```python
from build123d import *

# Parameters (mm, degrees)
SM_BASE_FLANGE_1_DEPTH = 351
SKETCH_6_W             = 30
SKETCH_6_H             = 25
CUT_EXTRUDE_1_DEPTH    = 3
SKETCH_7_R             = 2.5
CUT_EXTRUDE_1299_DEPTH = 569.507695638
SKETCH_8_R             = 3
CUT_EXTRUDE_1710_DEPTH = 1.5
SKETCH_10_W            = 65
SKETCH_10_H            = 25
CUT_EXTRUDE_4_DEPTH    = 3
OTHER_START            = -361.5
OTHER_1_DEPTH          = 723
SKETCH_11_R            = 10
CUT_EXTRUDE_2693_DEPTH = 10
SKETCH_12_R            = 4
CUT_EXTRUDE_3148_DEPTH = 10
SKETCH_13_R            = 2.5
SKETCH_13_R_2          = 5.5
CUT_EXTRUDE_3688_DEPTH = 10
SKETCH_15_R            = 14.5
SKETCH_15_R_2          = 2.5
CUT_EXTRUDE_4428_DEPTH = 1.5
SKETCH_16_R            = 2.5
CUT_EXTRUDE_5_DEPTH    = 10
SKETCH_17_W            = 100
SKETCH_17_H            = 10
CUT_EXTRUDE_6_DEPTH    = 10


# Read off the part's stored shape, not the designer's step: Затупленный угол1
# Sheet-metal steps are written as plain solids
with BuildPart() as part:
    # Sketch 1 → Базовая кромка1 (new, symmetric)
    with BuildSketch(Plane.XY):
        with BuildLine():
            Line((360, -175), (360, -197))
            ThreePointArc((360, -197), (360.878679656, -199.121320344), (363, -200))
            Line((363, -200), (397, -200))
            ThreePointArc((397, -200), (399.121320344, -199.121320344), (400, -197))
            Line((400, -197), (400, -3))
            ThreePointArc((400, -3), (399.121320344, -0.878679656), (397, 0))
            Line((397, 0), (-397, 0))
            ThreePointArc((-397, 0), (-399.121320344, -0.878679656), (-400, -3))
            Line((-400, -3), (-400, -197))
            ThreePointArc((-400, -197), (-399.121320344, -199.121320344), (-397, -200))
            Line((-397, -200), (-363, -200))
            ThreePointArc((-363, -200), (-360.878679656, -199.121320344), (-360, -197))
            Line((-360, -197), (-360, -175))
            Line((-360, -175), (-361.5, -175))
            Line((-361.5, -175), (-361.5, -197))
            ThreePointArc((-361.5, -197), (-361.939339828, -198.060660172), (-363, -198.5))
            Line((-363, -198.5), (-397, -198.5))
            ThreePointArc((-397, -198.5), (-398.060660172, -198.060660172), (-398.5, -197))
            Line((-398.5, -197), (-398.5, -3))
            ThreePointArc((-398.5, -3), (-398.060660172, -1.939339828), (-397, -1.5))
            Line((-397, -1.5), (397, -1.5))
            ThreePointArc((397, -1.5), (398.060660172, -1.939339828), (398.5, -3))
            Line((398.5, -3), (398.5, -197))
            ThreePointArc((398.5, -197), (398.060660172, -198.060660172), (397, -198.5))
            Line((397, -198.5), (363, -198.5))
            ThreePointArc((363, -198.5), (361.939339828, -198.060660172), (361.5, -197))
            Line((361.5, -197), (361.5, -175))
            Line((361.5, -175), (360, -175))
        make_face()
    extrude(amount=SM_BASE_FLANGE_1_DEPTH, both=True)

    # Эскиз6 → Вырез-Вытянуть1 (cut)
    with BuildSketch(Plane(origin=(-360, 0, 0), x_dir=(0, 0, -1), z_dir=(1, 0, 0))):
        with Locations((-336, -187.5)):
            Rectangle(SKETCH_6_W, SKETCH_6_H)
        with Locations((336, -187.5)):
            Rectangle(SKETCH_6_W, SKETCH_6_H)
    cut_extrude_1 = extrude(amount=-CUT_EXTRUDE_1_DEPTH, mode=Mode.SUBTRACT)

    # Зеркальное отражение1: Вырез-Вытянуть1 across plane
    add(cut_extrude_1.mirror(Plane(origin=(0, 0, 0), x_dir=(0, 0, 1), z_dir=(1, 0, 0))), mode=Mode.SUBTRACT)

    # Эскиз7 → Cut-Extrude 1299 (cut, through all)
    with BuildSketch(Plane.XZ.offset(200)):
        with Locations(Location((-388, 331, 0), (0, 0, 270))):
            Circle(SKETCH_7_R)
        with Locations(Location((-373, 341, 0), (0, 0, 270))):
            Circle(SKETCH_7_R)
        with Locations(Location((-373, -341, 0), (0, 0, 90))):
            Circle(SKETCH_7_R)
        with Locations(Location((-388, -331, 0), (0, 0, 90))):
            Circle(SKETCH_7_R)
        with Locations(Location((388, -331, 0), (0, 0, 270))):
            Circle(SKETCH_7_R)
        with Locations(Location((373, -341, 0), (0, 0, 270))):
            Circle(SKETCH_7_R)
        with Locations(Location((373, 341, 0), (0, 0, 270))):
            Circle(SKETCH_7_R)
        with Locations(Location((388, 331, 0), (0, 0, 270))):
            Circle(SKETCH_7_R)
    extrude(amount=-CUT_EXTRUDE_1299_DEPTH, mode=Mode.SUBTRACT)

    # Эскиз8 → Cut-Extrude 1710 (cut)
    with BuildSketch(Plane.XZ.offset(200)):
        with Locations(Location((371, 256.5, 0), (0, 0, 270))):
            Circle(SKETCH_8_R)
        with Locations(Location((371, 231.5, 0), (0, 0, 270))):
            Circle(SKETCH_8_R)
        with Locations(Location((371, -231.5, 0), (0, 0, 270))):
            Circle(SKETCH_8_R)
        with Locations(Location((371, -256.5, 0), (0, 0, 270))):
            Circle(SKETCH_8_R)
    extrude(amount=-CUT_EXTRUDE_1710_DEPTH, mode=Mode.SUBTRACT)

    # Эскиз10 → Вырез-Вытянуть4 (cut)
    with BuildSketch(Plane.ZY.offset(-360)):
        with Locations((-246, -187.5)):
            Rectangle(SKETCH_10_W, SKETCH_10_H)
        with Locations((246, -187.5)):
            Rectangle(SKETCH_10_W, SKETCH_10_H)
    cut_extrude_4 = extrude(amount=-CUT_EXTRUDE_4_DEPTH, mode=Mode.SUBTRACT)

    # Зеркальное отражение2: Вырез-Вытянуть4 across plane
    add(cut_extrude_4.mirror(Plane(origin=(0, 0, 0), x_dir=(0, 0, 1), z_dir=(1, 0, 0))), mode=Mode.SUBTRACT)

    # Other 1 outline → Other 1 (cut)
    with BuildSketch(Plane.YZ.offset(OTHER_START)):
        Polygon((-180, 213.5), (-175, 208.5), (-175, 213.5), align=None)
        Polygon((-175, -208.5), (-180, -213.5), (-175, -213.5), align=None)
        Polygon((-180, -278.5), (-175, -283.5), (-175, -278.5), align=None)
        Polygon((-175, 283.5), (-180, 278.5), (-175, 278.5), align=None)
    extrude(amount=OTHER_1_DEPTH, mode=Mode.SUBTRACT)

    # Эскиз11 → Cut-Extrude 2693 (cut)
    with BuildSketch(Plane(origin=(0, 0, 0), x_dir=(1, 0, 0), z_dir=(0, 1, 0))):
        with Locations(Location((365, 6, 0), (0, 0, 270))):
            Circle(SKETCH_11_R)
        with Locations(Location((365, 56, 0), (0, 0, 270))):
            Circle(SKETCH_11_R)
        with Locations(Location((285, 56, 0), (0, 0, 270))):
            Circle(SKETCH_11_R)
        with Locations(Location((285, 6, 0), (0, 0, 270))):
            Circle(SKETCH_11_R)
        with Locations(Location((-285, 6, 0), (0, 0, 90))):
            Circle(SKETCH_11_R)
        with Locations(Location((-285, 56, 0), (0, 0, 90))):
            Circle(SKETCH_11_R)
        with Locations(Location((-365, 56, 0), (0, 0, 90))):
            Circle(SKETCH_11_R)
        with Locations(Location((-365, 6, 0), (0, 0, 90))):
            Circle(SKETCH_11_R)
        with Locations(Location((365, -64, 0), (0, 0, 270))):
            Circle(SKETCH_11_R)
        with Locations(Location((-365, -64, 0), (0, 0, 90))):
            Circle(SKETCH_11_R)
    extrude(amount=-CUT_EXTRUDE_2693_DEPTH, mode=Mode.SUBTRACT)

    # Эскиз12 → Cut-Extrude 3148 (cut)
    with BuildSketch(Plane.XZ.offset(1.5)):
        with Locations(Location((325, -276, 0), (0, 0, 270))):
            Circle(SKETCH_12_R)
        with Locations(Location((325, 276, 0), (0, 0, 270))):
            Circle(SKETCH_12_R)
        with Locations(Location((-325, 276, 0), (0, 0, 270))):
            Circle(SKETCH_12_R)
        with Locations(Location((-325, -276, 0), (0, 0, 270))):
            Circle(SKETCH_12_R)
    extrude(amount=-CUT_EXTRUDE_3148_DEPTH, mode=Mode.SUBTRACT)

    # Эскиз13 → Cut-Extrude 3688 (cut)
    with BuildSketch(Plane.XZ.offset(1.5)):
        with Locations(Location((325, -151, 0), (0, 0, 270))):
            Circle(SKETCH_13_R)
        with Locations(Location((-325, -151, 0), (0, 0, 90))):
            Circle(SKETCH_13_R)
        with Locations(Location((325, -234.5, 0), (0, 0, 270))):
            Circle(SKETCH_13_R)
        with Locations(Location((-325, -234.5, 0), (0, 0, 270))):
            Circle(SKETCH_13_R)
        with Locations(Location((-325, 234.5, 0), (0, 0, 90))):
            Circle(SKETCH_13_R_2)
        with Locations(Location((325, 234.5, 0), (0, 0, 90))):
            Circle(SKETCH_13_R_2)
        with Locations(Location((-325, 151, 0), (0, 0, 270))):
            Circle(SKETCH_13_R_2)
        with Locations(Location((325, 151, 0), (0, 0, 90))):
            Circle(SKETCH_13_R_2)
    extrude(amount=-CUT_EXTRUDE_3688_DEPTH, mode=Mode.SUBTRACT)

    # Эскиз15 → Cut-Extrude 4428 (cut)
    with BuildSketch(Plane(origin=(0, 0, 0), x_dir=(1, 0, 0), z_dir=(0, 1, 0))):
        with Locations(Location((-360, -311, 0), (0, 0, 270))):
            Circle(SKETCH_15_R)
        with Locations(Location((-325, -311, 0), (0, 0, 270))):
            Circle(SKETCH_15_R)
        with Locations(Location((325, -311, 0), (0, 0, 90))):
            Circle(SKETCH_15_R)
        with Locations(Location((360, -311, 0), (0, 0, 90))):
            Circle(SKETCH_15_R)
        with Locations(Location((-290, -311, 0), (0, 0, 270))):
            Circle(SKETCH_15_R)
        with Locations(Location((290, -311, 0), (0, 0, 90))):
            Circle(SKETCH_15_R)
        with Locations(Location((-382.5, -311, 0), (0, 0, 270))):
            Circle(SKETCH_15_R_2)
        with Locations(Location((-267.5, -311, 0), (0, 0, 90))):
            Circle(SKETCH_15_R_2)
        with Locations(Location((382.5, -311, 0), (0, 0, 90))):
            Circle(SKETCH_15_R_2)
        with Locations(Location((267.5, -311, 0), (0, 0, 270))):
            Circle(SKETCH_15_R_2)
    extrude(amount=-CUT_EXTRUDE_4428_DEPTH, mode=Mode.SUBTRACT)

    # Эскиз16 → Вырез-Вытянуть5 (cut)
    with BuildSketch(Plane(origin=(-360, 0, 0), x_dir=(0, 0, -1), z_dir=(1, 0, 0))):
        with Locations((288.5, -185)):
            Circle(SKETCH_16_R)
        with Locations((308.5, -185)):
            Circle(SKETCH_16_R)
    cut_extrude_5 = extrude(amount=-CUT_EXTRUDE_5_DEPTH, mode=Mode.SUBTRACT)

    # Зеркальное отражение3: Вырез-Вытянуть5 across plane
    add(cut_extrude_5.mirror(Plane(origin=(0, 0, 0), x_dir=(0, 0, 1), z_dir=(1, 0, 0))), mode=Mode.SUBTRACT)

    # Эскиз17 → Вырез-Вытянуть6 (cut)
    with BuildSketch(Plane(origin=(-360, 0, 0), x_dir=(0, 0, -1), z_dir=(1, 0, 0))):
        with Locations((40, -188)):
            Rectangle(SKETCH_17_W, SKETCH_17_H)
    extrude(amount=-CUT_EXTRUDE_6_DEPTH, mode=Mode.SUBTRACT)


solid = part.part
```
Design review of the part built by this model. Coordinates are the model's own, in mm. A direction names the side the tool comes from. Round coordinates to 2 decimals unless told otherwise and drop trailing zeros. Order: outer loops, then holes, each group sorted by start corner. A loop starts at its lowest first (then second) coordinate and runs counter-clockwise, first axis right, second up. Notation, with made-up numbers: (89.5, -7.5) - (97.5, -7.5) arc R26 ccw to (97.5, 6.5) - close; hole circle Ø9 at (79.25, 12.25). An arc over 180 degrees is marked (long way). One line per question, with ' | ' between items.
Item 1: Take a section at C-C, the plane z = 134. Write out the cut boundary in (x, y), then the cut area to 3 significant figures.
Checks:
outline: (-400, -197) arc R3 ccw to (-397, -200) - (-363, -200) arc R3 ccw to (-360, -197) - (-360, -175) - (-361.5, -175) - (-361.5, -197) arc R1.5 cw to (-363, -198.5) - (-397, -198.5) arc R1.5 cw to (-398.5, -197) - (-398.5, -3) arc R1.5 cw to (-397, -1.5) - (397, -1.5) arc R1.5 cw to (398.5, -3) - (398.5, -197) arc R1.5 cw to (397, -198.5) - (363, -198.5) arc R1.5 cw to (361.5, -197) - (361.5, -175) - (360, -175) - (360, -197) arc R3 ccw to (363, -200) - (397, -200) arc R3 ccw to (400, -197) - (400, -3) arc R3 ccw to (397, 0) - (-397, 0) arc R3 ccw to (-400, -3) - close | area: 1,970 mm²
Item 2: Take a section at D-D, the plane x = 7. Write out the cut boundary in (y, z), then the cut area to 3 significant figures.
Checks:
outline: (-1.5, -351) - (0, -351) - (0, 351) - (-1.5, 351) - close | area: 1,050 mm²
Item 3: Machinability: for faces 1 (the face through (-380, -198.5, 5)), 2 (the face through (-374.915, -0.74, -54.698)), 3 (the face through (-360, -186, 300)), which of the approach directions +Z, -Z, +X, -X, +Y, -Y give a long, thin tool a straight path to every point of the face, cutting with its end or side? Answer none if there is none.
Checks:
face 1: +Z, -Z | face 2: +Y | face 3: +Z, -Z, -Y
Item 4: Take a section at B-B, the plane y = -61.5. Write out the cut boundary in (x, z), then the cut area to 3 significant figures.
Checks:
outline: (-400, -351) - (-398.5, -351) - (-398.5, 351) - (-400, 351) - close; (398.5, -351) - (400, -351) - (400, 351) - (398.5, 351) - close | area: 2,110 mm²
Item 5: Wall thickness on line 1 (X direction, y = -179.5, z = -47); line 2 (Z direction, x = 361, y = -185); line 3 (X direction, y = -199.6, z = -231.5): over which ranges is each line inside the solid? List them lowest first. Write a range as [from, to].
Checks:
line 1: [-400, -398.5], [-361.5, -360], [360, 361.5], [398.5, 400] | line 2: [-321, -311], [-306, -291], [-286, -278.5], [-213.5, 213.5], [278.5, 321] | line 3: [-398.5, -363], [363, 368], [374, 398.5]
Item 6: Draft analysis for pull direction Y (two halves, no side actions). For faces 4 (the face through (-361.5, -186, -299)), 5 (the face through (-380, -200, 5)), 6 (the face through (276.128, -0.74, -1.386)), state which applies: +Y half, -Y half, draft (parallel to the pull), parting line (faces both ways), or undercut.
Checks:
face 4: undercut | face 5: -Y half | face 6: draft
Item 7: For P1, Ø5, axis at x = 371, z = -256.5, coming from the -Y side; P2, Ø0.9, axis at x = 361, y = -183.5, coming from the -Z side; P3, Ø0.9, axis at x = 361, y = -185, coming from the +Z side, all flat-tipped, find the tip position at first contact; note any pin that passes through.
Checks:
P1: y = -1.5 | P2: z = -321 | P3: z = 321
